Design review of the part built by this model. Coordinates are the model's own, in mm. Give positions to 0.01 mm unless a question says otherwise; leave off trailing zeros. Loops run counter-clockwise (first coordinate to the right, second up) from the corner with the lowest first, then second, coordinate; pieces in that order, holes last. Notation, with made-up numbers: (37, 19.5) - (85, 19.5) arc R10 ccw to (85, 37.5) - close; hole circle Ø3 at (-20, 16.5). An arc over 180 degrees is marked (long way). Write each question's results on one line, items separated by ' | '.
Autodesk Inventor part; units mm, degrees
ref_plane "YZ Plane" through (0, 0, 0) normal (1, 0, 0) x (0, 1, 0)
ref_plane "XZ Plane" through (0, 0, 0) normal (0, 1, 0) x (-1, 0, 0)
ref_plane "XY Plane" through (0, 0, 0) normal (0, 0, 1) x (1, 0, 0)
sketch "Náčrt6" plane through (0, 0, 0) normal (0, 0, 1) x (1, 0, 0)
  line L0 (0, 10) -> (1200, 331.539)
  line L1 (0, 10) -> (0, 0)
  line L2 (0, -10) -> (1200, -331.539)
  line L3 (1200, 331.539) -> (1200, 0)
  line L4 (0, 0) -> (1200, 0) construction
  line L5 (1200, 0) -> (1200, -331.539)
  line L6 (0, 0) -> (0, -10)
  dimension "d15" = 20
  dimension "d16" = 30
  dimension "d17" = 1200
extrude "Vysunutí3" add sketch "Náčrt6" along normal mid plane 20
sketch "Náčrt7" plane through (0, -10, 10) normal (-1, 0, 0) x (0, 0, 1)
  circle A0 centre (-10, 10) radius 5
  dimension "d22" = 10
extrude "Vysunutí4" cut sketch "Náčrt7" against normal blind 20
properties part number "Pieskovy_luc"
Item 1: We need section B-B on y = 43. Give the boundary of the cut face in (x, z), then the cut area to 3 significant figures.
Output values:
outline: (123.16, -10) - (1200, -10) - (1200, 10) - (123.16, 10) - close | area: 21,500 mm²
Item 2: We need section C-C on x = 625.5. Give the boundary of the cut face in (y, z), then the cut area to 3 significant figures.
Output values:
outline: (-177.6, -10) - (177.6, -10) - (177.6, 10) - (-177.6, 10) - close | area: 7,100 mm²
Item 3: Clearance check with flat-ended pins moving along their axes: P1, Ø5, axis at x = 796, z = -5, coming from the -Y side; P2, Ø3, axis at y = -0.5, z = -1.5, coming from the -X side; P3, Ø10, axis at x = 950, z = -7, coming from the +Y side. State where each tip first meets the part, or that it passes through.
Output values:
P1: stops at y = -223.96 | P2: stops at x = 20 | P3: stops at y = 265.89
Item 4: We need section A-A on z = 0. Give the boundary of the cut face in (x, y).
Output values:
outline: (0, -10) - (1200, -331.54) - (1200, 331.54) - (0, 10) - (0, 5) - (20, 5) - (20, -5) - (0, -5) - close
Item 5: Wall thickness on probe 1 along Y at (x, z) = (9, 0); probe 2 along Y at (x, z) = (9.5, 0); probe 3 along Y at (x, z) = (99, -2): over which ranges is each line inside the solid? List them lowest first.
Output values:
probe 1: y = -12.41 to -5, 5 to 12.41 | probe 2: y = -12.55 to -5, 5 to 12.55 | probe 3: y = -36.53 to 36.53
